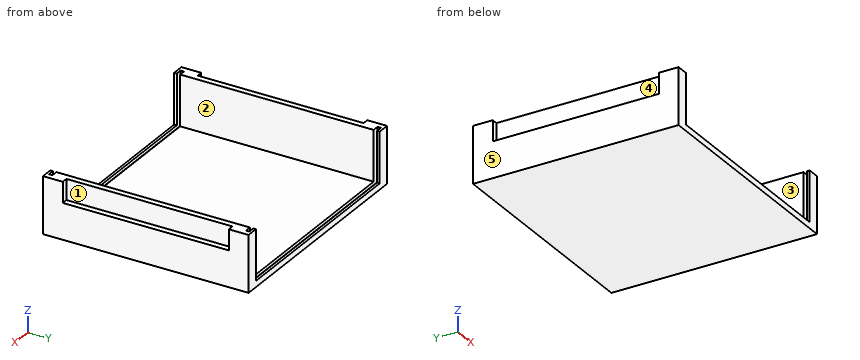
```python
from build123d import *

# Parameters (mm, degrees)
SKETCH_W        = 114
SKETCH_H        = 102
PAD_DEPTH       = 3
SKETCH001_W     = 6
SKETCH001_H     = 102
PAD001_DEPTH    = 25
SKETCH002_W     = 6
SKETCH002_H     = 102
PAD002_DEPTH    = 25
SKETCH003_W     = 82.4
SKETCH003_H     = 10.2
POCKET_DEPTH    = 3
SKETCH004_W     = 82.4
SKETCH004_H     = 10.2
POCKET001_DEPTH = 3
SKETCH005_W     = 1.7
SKETCH005_H     = 25
POCKET002_DEPTH = 3.2
SKETCH006_W     = 102
SKETCH006_H     = 1.7
POCKET003_DEPTH = 1.6
SKETCH007_W     = 3.2
SKETCH007_H     = 1.7
POCKET004_DEPTH = 1.6
SKETCH008_W     = 1.7
SKETCH008_H     = 25
POCKET005_DEPTH = 3.2
SKETCH010_W     = 3.2
SKETCH010_H     = 1.7
POCKET006_DEPTH = 1.6
SKETCH011_W     = 1.7
SKETCH011_H     = 25
POCKET007_DEPTH = 3.2
SKETCH012_W     = 102
SKETCH012_H     = 1.7
POCKET008_DEPTH = 1.6
SKETCH013_W     = 3.2
SKETCH013_H     = 1.7
POCKET009_DEPTH = 1.6
SKETCH014_W     = 1.7
SKETCH014_H     = 25
POCKET010_DEPTH = 3.2
SKETCH015_W     = 3.2
SKETCH015_H     = 1.7
POCKET011_DEPTH = 1.6


with BuildPart() as part:
    # Sketch → Pad (new body)
    with BuildSketch(Plane.XY):
        with Locations((57, -51)):
            Rectangle(SKETCH_W, SKETCH_H)
    extrude(amount=PAD_DEPTH)

    # Sketch001 (on Face6 of Pad) → Pad001 (join)
    with BuildSketch(Plane.XY.offset(3)):
        with Locations((3, -51)):
            Rectangle(SKETCH001_W, SKETCH001_H)
    extrude(amount=PAD001_DEPTH)

    # Sketch002 (on Face6 of Pad001) → Pad002 (join)
    with BuildSketch(Plane.XY.offset(3)):
        with Locations((111, -51)):
            Rectangle(SKETCH002_W, SKETCH002_H)
    extrude(amount=PAD002_DEPTH)

    # Sketch003 (on Face10 of Pad002) → Pocket (cut)
    with BuildSketch(Plane.YZ.offset(114)):
        with Locations((-51, 22.9)):
            Rectangle(SKETCH003_W, SKETCH003_H)
    extrude(amount=-POCKET_DEPTH, mode=Mode.SUBTRACT)

    # Sketch004 (on Face9 of Pocket) → Pocket001 (cut)
    with BuildSketch(Plane(origin=(0, 0, 0), x_dir=(0, -1, 0), z_dir=(-1, 0, 0))):
        with Locations((51, 22.9)):
            Rectangle(SKETCH004_W, SKETCH004_H)
    extrude(amount=-POCKET001_DEPTH, mode=Mode.SUBTRACT)

    # Sketch005 (on Face11 of Pocket001) → Pocket002 (cut)
    with BuildSketch(Plane.YZ.offset(6)):
        with Locations((-99.85, 15.5)):
            Rectangle(SKETCH005_W, SKETCH005_H)
    extrude(amount=-POCKET002_DEPTH, mode=Mode.SUBTRACT)

    # Sketch006 (on Face6 of Pocket002) → Pocket003 (cut)
    with BuildSketch(Plane.XY.offset(3)):
        with Locations((57, -99.85)):
            Rectangle(SKETCH006_W, SKETCH006_H)
    extrude(amount=-POCKET003_DEPTH, mode=Mode.SUBTRACT)

    # Sketch007 (on Face35 of Pocket003) → Pocket004 (cut)
    with BuildSketch(Plane.XY.offset(3)):
        with Locations((4.4, -99.85)):
            Rectangle(SKETCH007_W, SKETCH007_H)
    extrude(amount=-POCKET004_DEPTH, mode=Mode.SUBTRACT)

    # Sketch008 (on Face13 of Pocket004) → Pocket005 (cut)
    with BuildSketch(Plane(origin=(108, 0, 0), x_dir=(0, -1, 0), z_dir=(-1, 0, 0))):
        with Locations((99.85, 15.5)):
            Rectangle(SKETCH008_W, SKETCH008_H)
    extrude(amount=-POCKET005_DEPTH, mode=Mode.SUBTRACT)

    # Sketch010 (on Face41 of Pocket005) → Pocket006 (cut)
    with BuildSketch(Plane.XY.offset(3)):
        with Locations((109.6, -99.85)):
            Rectangle(SKETCH010_W, SKETCH010_H)
    extrude(amount=-POCKET006_DEPTH, mode=Mode.SUBTRACT)

    # Sketch011 (on Face11 of Pocket006) → Pocket007 (cut)
    with BuildSketch(Plane.YZ.offset(6)):
        with Locations((-2.15, 15.5)):
            Rectangle(SKETCH011_W, SKETCH011_H)
    extrude(amount=-POCKET007_DEPTH, mode=Mode.SUBTRACT)

    # Sketch012 (on Face6 of Pocket007) → Pocket008 (cut)
    with BuildSketch(Plane.XY.offset(3)):
        with Locations((57, -2.15)):
            Rectangle(SKETCH012_W, SKETCH012_H)
    extrude(amount=-POCKET008_DEPTH, mode=Mode.SUBTRACT)

    # Sketch013 (on Face44 of Pocket008) → Pocket009 (cut)
    with BuildSketch(Plane.XY.offset(3)):
        with Locations((4.4, -2.15)):
            Rectangle(SKETCH013_W, SKETCH013_H)
    extrude(amount=-POCKET009_DEPTH, mode=Mode.SUBTRACT)

    # Sketch014 (on Face13 of Pocket009) → Pocket010 (cut)
    with BuildSketch(Plane(origin=(108, 0, 0), x_dir=(0, -1, 0), z_dir=(-1, 0, 0))):
        with Locations((2.15, 15.5)):
            Rectangle(SKETCH014_W, SKETCH014_H)
    extrude(amount=-POCKET010_DEPTH, mode=Mode.SUBTRACT)

    # Sketch015 (on Face53 of Pocket010) → Pocket011 (cut)
    with BuildSketch(Plane.XY.offset(3)):
        with Locations((109.6, -2.15)):
            Rectangle(SKETCH015_W, SKETCH015_H)
    extrude(amount=-POCKET011_DEPTH, mode=Mode.SUBTRACT)


solid = part.part
```
Part model, mm, in its own coordinate system. Face numbers are marked on the shaded views. A direction names the side the tool comes from. Round coordinates to 2 decimals unless told otherwise and drop trailing zeros. Order: outer loops, then holes, each group sorted by start corner. A loop starts at its lowest first (then second) coordinate and runs counter-clockwise, first axis right, second up. Notation, with made-up numbers: M 10,43 L 28,43 A17 ccw 28,71 Z; hole C 73,74.25 d11. An arc over 180 degrees is marked long. Put each result on its own line as item: value. Start each with the question number.
1. Tool access for the marked faces 3, 4 and 5: list every direction of +Z, -Z, +X, -X, +Y, -Y with a clear straight run to the whole face (end or side of a thin tool).
2. Drop flat-ended pins along their axis: pin 1 (0.9 mm diameter, centred on x = 2, z = 24, fed in from +Y); pin 2 (5 mm diameter, centred on x = 57.5, y = -81.5, fed in from +Z); pin 3 (8 mm diameter, centred on y = -34, z = 25, fed in from -X); pin 4 (10 mm diameter, centred on x = 46, z = 10.5, fed in from +Y). Give the stop position or say it passes through.
3. Slice it at A-A on z = 14. List the corners of the cut face in (x, y).
4. Slice it at B-B on y = -14. List the corners of the cut face in (x, z).
5. Two-plate mould, pull along Y, no slides. Class the marked faces 1 and 2: +Y half, -Y half, draft (parallel to the pull), parting line (faces both ways), or undercut.
6. Slice it at C-C on x = 78. List the corners of the cut face in (y, z), then the cut area to 3 significant figures.
7. Drill centre lines: probe 1 along X at (y, z) = (-32.5, 18.5); probe 2 along X at (y, z) = (-26.5, 6.25); probe 3 along Z at (x, y) = (35, -84.5). Where is each one in solid material? Low to high. Write a range as [from, to].
Findings:
1. face 3: +Z, +Y, -Y
1. face 4: +Z, -X
1. face 5: +Z, -Z, -X, +Y, -Y
2. pin 1: y = 0
2. pin 2: z = 3
2. pin 3: x = 3
2. pin 4: through
3. outline: M 0,-102 L 6,-102 L 6,-100.7 L 2.8,-100.7 L 2.8,-99 L 6,-99 L 6,-3 L 2.8,-3 L 2.8,-1.3 L 6,-1.3 L 6,0 L 0,0 Z; M 108,-102 L 114,-102 L 114,0 L 108,0 L 108,-1.3 L 111.2,-1.3 L 111.2,-3 L 108,-3 L 108,-99 L 111.2,-99 L 111.2,-100.7 L 108,-100.7 Z
4. outline: M 0,0 L 114,0 L 114,17.8 L 111,17.8 L 111,28 L 108,28 L 108,3 L 6,3 L 6,28 L 3,28 L 3,17.8 L 0,17.8 Z
5. face 1: undercut
5. face 2: draft
6. outline: M -102,0 L 0,0 L 0,3 L -1.3,3 L -1.3,1.4 L -3,1.4 L -3,3 L -99,3 L -99,1.4 L -100.7,1.4 L -100.7,3 L -102,3 Z
6. area: 301 mm2
7. probe 1: [3, 6], [108, 111]
7. probe 2: [0, 6], [108, 114]
7. probe 3: [0, 3]
